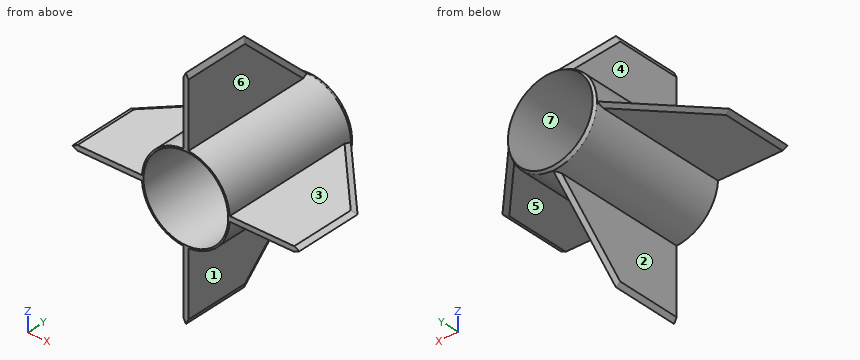
```python
from build123d import *

# Parameters (mm, degrees)
SKETCH1_R                                     = 35.27
SKETCH1_R_2                                   = 34
BOSS_EXTRUDE1_DEPTH                           = 115.6
SKETCH3_W                                     = 4.08
SKETCH3_H                                     = 113.06
BOSS_EXTRUDE2_DEPTH                           = 90.984
CUT_EXTRUDE1_DEPTH                            = 152.767863384
CUT_EXTRUDE4_DEPTH                            = 152.279281979
MIRROR4_AT_THE_SECOND_PLANE_COPY_1_DEPTH      = 152.279281979
CUT_EXTRUDE5_REACH                            = 175.905
CUT_EXTRUDE5_END_RADIUS                       = 35.27
MIRROR5_AT_THE_SECOND_PLANE_COPY_1_REACH      = 175.905
MIRROR5_AT_THE_SECOND_PLANE_COPY_1_END_RADIUS = 35.27
SKETCH12_W                                    = 4.08
SKETCH12_H                                    = 113.06
BOSS_EXTRUDE3_DEPTH                           = 90.984
CUT_EXTRUDE6_DEPTH                            = 175.054338734
CUT_EXTRUDE7_DEPTH                            = 173.972646716
MIRROR6_START                                 = -1
MIRROR6_DEPTH                                 = 114.06
MIRROR6_START_2                               = -2.04
MIRROR6_2_DEPTH                               = 4.08
MIRROR6_START_3                               = 40.689281773
MIRROR6_3_OUTLINE_W                           = 8
MIRROR6_3_OUTLINE_H                           = 61
MIRROR6_3_DEPTH                               = 3.310718227
CUT_EXTRUDE8_REACH                            = 195.073
CUT_EXTRUDE8_END_RADIUS                       = 35.27
MIRROR7_AT_THE_SECOND_PLANE_COPY_1_REACH      = 195.073
MIRROR7_AT_THE_SECOND_PLANE_COPY_1_END_RADIUS = 35.27
CUT_EXTRUDE9_DEPTH                            = 173.972646716
CUT_EXTRUDE9_DEPTH_BACK                       = 173.972646716
SKETCH17_R                                    = 34
SCALE2_SCALE                                  = 0.985294118


with BuildPart() as part:
    # Sketch1 → Boss-Extrude1 (new body)
    with BuildSketch(Plane(origin=(0, 0, 0), x_dir=(1, 0, 0), z_dir=(0, 1, 0))):
        with Locations(Location((0, 0, 0), (0, 0, 270))):
            Circle(SKETCH1_R)
        with Locations(Location((0, 0, 0), (0, 0, 270))):
            Circle(SKETCH1_R_2, mode=Mode.SUBTRACT)
    extrude(amount=BOSS_EXTRUDE1_DEPTH)

    # Sketch2 → Cut-Revolve3 (revolve, cut)
    with BuildSketch(Plane(origin=(0, 0, 0), x_dir=(0, 0, -1), z_dir=(1, 0, 0))):
        Polygon((-35.27, 113.06), (-35.27, 115.6), (-34, 115.6), align=None)
    revolve(axis=Axis((0, 115.6, 0), (0, -1, 0)), mode=Mode.SUBTRACT)

    # Sketch3 → Boss-Extrude2 (add, symmetric)
    with BuildSketch(Plane.XY):
        with Locations((0, 56.53)):
            Rectangle(SKETCH3_W, SKETCH3_H)
    extrude(amount=BOSS_EXTRUDE2_DEPTH, both=True)

    # Sketch4 → Cut-Extrude1 (cut, symmetric)
    with BuildSketch(Plane.ZY.offset(2.04)):
        Polygon((35.210954261, 113.06), (90.984, 54.4), (90.984, 113.06), align=None)
    cut_extrude1 = extrude(amount=CUT_EXTRUDE1_DEPTH, both=True, mode=Mode.SUBTRACT)

    # Mirror3: Cut-Extrude1 across plane
    add(cut_extrude1.mirror(Plane.XY), mode=Mode.SUBTRACT)

    # Sketch7 → Cut-Extrude4 (cut, symmetric)
    with BuildSketch(Plane.XZ):
        Polygon((0, 90.984), (-2.04, 86.904), (-2.04, 90.984), align=None)
    cut_extrude4 = extrude(amount=CUT_EXTRUDE4_DEPTH, both=True, mode=Mode.SUBTRACT)

    # Mirror4: Cut-Extrude4 across plane
    add(cut_extrude4.mirror(Plane(origin=(0, 0, 0), x_dir=(0, 0, 1), z_dir=(1, 0, 0))), mode=Mode.SUBTRACT)

    # Mirror4 at the second plane: Cut-Extrude4 across plane
    add(cut_extrude4.mirror(Plane.XY), mode=Mode.SUBTRACT)

    # Mirror4 at the second plane copy 1 sketc → Mirror4 at the second plane copy 1 (cut, symmetric)
    with BuildSketch(Plane(origin=(0, 0, 0), x_dir=(-1, 0, 0), z_dir=(0, -1, 0))):
        Polygon((0, 90.984), (-2.04, 86.904), (-2.04, 90.984), align=None)
    extrude(amount=MIRROR4_AT_THE_SECOND_PLANE_COPY_1_DEPTH, both=True, mode=Mode.SUBTRACT)

    # Cut-Extrude5: up to this cylinder (the profile starts outside it)
    cut_extrude5_end = Plane(origin=(0, 53.462894, 0), z_dir=(0, -1, 0)) * Cylinder(CUT_EXTRUDE5_END_RADIUS, 423.35, mode=Mode.PRIVATE)
    # Sketch11 → Cut-Extrude5 (cut, up to the surface)
    with BuildSketch(Plane(origin=(0, -16.862580362, -16.032687791), x_dir=(1, 0, 0), z_dir=(0, 0.7247153095275539, 0.6890484163949453)), mode=Mode.PRIVATE) as cut_extrude5_sk1:
        Polygon((0, 103.421731574), (-2.04, 103.421731574), (-2.04, 99.341731574), align=None)
    cut_extrude5_tool1 = extrude(cut_extrude5_sk1.sketch, amount=CUT_EXTRUDE5_REACH, mode=Mode.PRIVATE) - cut_extrude5_end
    cut_extrude5 = cut_extrude5_tool1.solids().sort_by_distance((-1.36, 53.462894, -89.998387))[0]
    add(cut_extrude5, mode=Mode.SUBTRACT)

    # Mirror5: Cut-Extrude5 across plane
    add(cut_extrude5.mirror(Plane(origin=(0, 0, 0), x_dir=(0, 0, 1), z_dir=(1, 0, 0))), mode=Mode.SUBTRACT)

    # Mirror5 at the second plane: Cut-Extrude5 across plane
    add(cut_extrude5.mirror(Plane.XY), mode=Mode.SUBTRACT)

    # Mirror5 at the second plane copy 1: up to this cylinder (the profile starts outside it)
    mirror5_at_the_second_plane_copy_1_end = Plane(origin=(0, 53.462894, 0), z_dir=(0, -1, 0)) * Cylinder(MIRROR5_AT_THE_SECOND_PLANE_COPY_1_END_RADIUS, 423.35, mode=Mode.PRIVATE)
    # Mirror5 at the second plane copy 1 sketc → Mirror5 at the second plane copy 1 (cut, up to the surface)
    with BuildSketch(Plane(origin=(0, -16.862580362, 16.032687791), x_dir=(-1, 0, 0), z_dir=(0, 0.7247153095275539, -0.6890484163949453)), mode=Mode.PRIVATE) as mirror5_at_the_second_plane_copy_1_sk1:
        Polygon((0, 103.421731574), (-2.04, 103.421731574), (-2.04, 99.341731574), align=None)
    mirror5_at_the_second_plane_copy_1_tool1 = extrude(mirror5_at_the_second_plane_copy_1_sk1.sketch, amount=MIRROR5_AT_THE_SECOND_PLANE_COPY_1_REACH, mode=Mode.PRIVATE) - mirror5_at_the_second_plane_copy_1_end
    add(mirror5_at_the_second_plane_copy_1_tool1.solids().sort_by_distance((-1.36, 53.462894, -89.998387))[0], mode=Mode.SUBTRACT)

    # Sketch12 → Boss-Extrude3 (add, symmetric)
    with BuildSketch(Plane(origin=(0, 0, 0), x_dir=(0, 0, -1), z_dir=(1, 0, 0))):
        with Locations((0, 56.53)):
            Rectangle(SKETCH12_W, SKETCH12_H)
    extrude(amount=BOSS_EXTRUDE3_DEPTH, both=True)

    # Sketch13 → Cut-Extrude6 (cut, through all)
    with BuildSketch(Plane.XY.offset(2.04)):
        Polygon((35.210954261, 113.06), (90.984, 113.06), (90.984, 54.4), align=None)
    extrude(amount=-CUT_EXTRUDE6_DEPTH, mode=Mode.SUBTRACT)

    # Sketch14 → Cut-Extrude7 (cut, through all)
    with BuildSketch(Plane.XZ):
        Polygon((90.984, 0), (90.984, 2.04), (86.904, 2.04), align=None)
    extrude(amount=-CUT_EXTRUDE7_DEPTH, mode=Mode.SUBTRACT)

    # Mirror6: read off the stored shape, not the designer's step
    # Mirror6 outline → Mirror6 (cut)
    with BuildSketch(Plane(origin=(0, 0, 0), x_dir=(1, 0, 0), z_dir=(0, 1, 0)).offset(MIRROR6_START)):
        Polygon((-90.984, 2.04), (-90.984, 0), (-86.904, 2.04), align=None)
        Polygon((-86.904, -2.04), (-90.984, 0), (-90.984, -2.04), align=None)
    extrude(amount=MIRROR6_DEPTH, mode=Mode.SUBTRACT)

    # Mirror6 2 outline → Mirror6 2 (cut)
    with BuildSketch(Plane.XY.offset(MIRROR6_START_2)):
        Polygon((-90.984, 54.4), (-35.210954261, 113.06), (-92, 113.06), (-92, 53.331409264), align=None)
    extrude(amount=MIRROR6_2_DEPTH, mode=Mode.SUBTRACT)

    # Mirror6 3 outline → Mirror6 3 (cut)
    with BuildSketch(Plane(origin=(0, 0, 0), x_dir=(0.8944271909999159, 0, 0.44721359549995804), z_dir=(0.447213595499958, 0, -0.894427190999916)).offset(MIRROR6_START_3)):
        with Locations((79, -29.5)):
            Rectangle(MIRROR6_3_OUTLINE_W, MIRROR6_3_OUTLINE_H)
    extrude(amount=MIRROR6_3_DEPTH, mode=Mode.SUBTRACT)

    # Cut-Extrude8: up to this cylinder (the profile starts outside it)
    cut_extrude8_end = Plane(origin=(0, 53.462894, 0), z_dir=(0, -1, 0)) * Cylinder(CUT_EXTRUDE8_END_RADIUS, 461.686, mode=Mode.PRIVATE)
    # Sketch15 → Cut-Extrude8 (cut, up to the surface)
    with BuildSketch(Plane(origin=(16.032687791, -16.862580362, 0), x_dir=(0.7247153095275543, 0.6890484163949449, 0), z_dir=(-0.6890484163949449, 0.7247153095275543, 0)), mode=Mode.PRIVATE) as cut_extrude8_sk1:
        Polygon((103.421731574, 0), (103.421731574, 2.04), (99.341731574, 2.04), align=None)
    cut_extrude8_tool1 = extrude(cut_extrude8_sk1.sketch, amount=CUT_EXTRUDE8_REACH, mode=Mode.PRIVATE) - cut_extrude8_end
    cut_extrude8 = cut_extrude8_tool1.solids().sort_by_distance((89.998387, 53.462894, -1.36))[0]
    add(cut_extrude8, mode=Mode.SUBTRACT)

    # Mirror7: Cut-Extrude8 across plane
    add(cut_extrude8.mirror(Plane(origin=(0, 0, 0), x_dir=(0, 0, 1), z_dir=(1, 0, 0))), mode=Mode.SUBTRACT)

    # Mirror7 at the second plane: Cut-Extrude8 across plane
    add(cut_extrude8.mirror(Plane.XY), mode=Mode.SUBTRACT)

    # Mirror7 at the second plane copy 1: up to this cylinder (the profile starts outside it)
    mirror7_at_the_second_plane_copy_1_end = Plane(origin=(0, 53.462894, 0), z_dir=(0, -1, 0)) * Cylinder(MIRROR7_AT_THE_SECOND_PLANE_COPY_1_END_RADIUS, 461.686, mode=Mode.PRIVATE)
    # Mirror7 at the second plane copy 1 sketc → Mirror7 at the second plane copy 1 (cut, up to the surface)
    with BuildSketch(Plane(origin=(-16.032687791, -16.862580362, 0), x_dir=(-0.7247153095275543, 0.6890484163949449, 0), z_dir=(0.6890484163949449, 0.7247153095275543, 0)), mode=Mode.PRIVATE) as mirror7_at_the_second_plane_copy_1_sk1:
        Polygon((103.421731574, 0), (103.421731574, 2.04), (99.341731574, 2.04), align=None)
    mirror7_at_the_second_plane_copy_1_tool1 = extrude(mirror7_at_the_second_plane_copy_1_sk1.sketch, amount=MIRROR7_AT_THE_SECOND_PLANE_COPY_1_REACH, mode=Mode.PRIVATE) - mirror7_at_the_second_plane_copy_1_end
    add(mirror7_at_the_second_plane_copy_1_tool1.solids().sort_by_distance((89.998387, 53.462894, -1.36))[0], mode=Mode.SUBTRACT)

    # Sketch17 → Cut-Extrude9 (cut, two sides: drawn at the far end of the back side and taken through both)
    with BuildSketch(Plane.XZ.offset(-CUT_EXTRUDE9_DEPTH_BACK)):
        with Locations(Location((0, 0, 0), (0, 0, 90))):
            Circle(SKETCH17_R)
    extrude(amount=CUT_EXTRUDE9_DEPTH + CUT_EXTRUDE9_DEPTH_BACK, mode=Mode.SUBTRACT)


with BuildPart() as part_1:
    # Scale2: scaled about (0, 47.022865963, 0)
    add(part.part.scale(SCALE2_SCALE).moved(Location((0, 0.691512735, 0))))


solid = part_1.part
```
Verification items for the finished model (mm, model axes). Face numbers are marked on the shaded views. A direction names the side the tool comes from. Give positions to 0.01 mm unless a question says otherwise; leave off trailing zeros. Order: outer loops, then holes, each group sorted by start corner. A loop starts at its lowest first (then second) coordinate and runs counter-clockwise, first axis right, second up. Notation, with made-up numbers: M 47,88 L 99,88 A34 cw 99,124 Z; hole C -27,-9 d11. An arc over 180 degrees is marked long. Return JSON: item names as keys, results as strings. Group by question number.
1) Section check A-A on y = 50. Record the cut outline in (x, z), and give its area (3 significant figures).
2) Section check C-C on z = 66. Record the cut outline in (x, y).
3) Go/stop test with flat-tipped pins: pin 1 Ø1 at (y, z) = (37, 28) entering from -X; pin 2 Ø4 at (x, y) = (16.5, 27) entering from +Z; pin 3 Ø1 at (x, y) = (-42, 66) entering from -Z. Record where each tip stops, or that it passes through.
4) Scan lines: line 1 (X direction, y = 31, z = 0); line 2 (Z direction, x = 69.5, y = 36.5); line 3 (X direction, y = 80.5, z = -11). Record each from-to range of solid material in increasing order.
5) Section check B-B on x = 53. Record the cut outline in (y, z), and give its area (3 significant figures).
6) Section check D-D on y = 91.5. Record the cut outline in (x, z).
7) Access from +Z, -Z, +X, -X, +Y, -Y to the whole of each face (thin tool, end or side, straight path). Record for the marked faces 1, 2, 3 and 4.
8) Mould release check, pull along Z, two halves, no side actions. Record for the marked faces 5, 6 and 7: pulls with the +Z half, pulls with the -Z half, needs draft (parallel to the pull), parting line crosses it, or undercut.
Answer block:
{
 "1": {"outline": "M -89.65,0 L -85.63,-2.01 L -34.69,-2.01 A34.75 ccw -2.01,-34.69 L -2.01,-85.63 L 0,-89.65 L 2.01,-85.63 L 2.01,-34.69 A34.75 ccw 34.69,-2.01 L 85.63,-2.01 L 89.65,0 L 85.63,2.01 L 34.69,2.01 A34.75 ccw 2.01,34.69 L 2.01,85.63 L 0,89.65 L -2.01,85.63 L -2.01,34.69 A34.75 ccw -34.69,2.01 L -85.63,2.01 Z; hole C 0,0 d67", "area": "1,120 mm^2"},
 "2": {"outline": "M -2.01,0.69 L 2.01,0.69 L 2.01,73.33 L 0,79.16 L -2.01,73.33 Z"},
 "3": {"pin 1": "stops at x = -21.25", "pin 2": "stops at z = 31.58", "pin 3": "stops at z = -2.01"},
 "4": {"line 1": "x = -89.65 to -33.5, 33.5 to 89.65", "line 2": "z = -2.01 to 2.01", "line 3": "x = -32.96 to -31.64, 31.64 to 32.96"},
 "5": {"outline": "M 0.69,-2.01 L 87,-2.01 L 92.83,0 L 87,2.01 L 0.69,2.01 Z", "area": "359 mm^2"},
 "6": {"outline": "M -54.27,0 L -48.72,-2.01 L -34.69,-2.01 A34.75 ccw -2.01,-34.69 L -2.01,-48.72 L 0,-54.27 L 2.01,-48.72 L 2.01,-34.69 A34.75 ccw 34.69,-2.01 L 48.72,-2.01 L 54.27,0 L 48.72,2.01 L 34.69,2.01 A34.75 ccw 2.01,34.69 L 2.01,48.72 L 0,54.27 L -2.01,48.72 L -2.01,34.69 A34.75 ccw -34.69,2.01 L -48.72,2.01 Z; hole C 0,0 d67"},
 "7": {"face 1": "-Z, +X, +Y, -Y", "face 2": "-Z, -X, +Y, -Y", "face 3": "+Z, +X, +Y, -Y", "face 4": "+Z, -X, +Y, -Y"},
 "8": {"face 5": "pulls with the -Z half", "face 6": "needs draft", "face 7": "undercut"}
}
